Input: part model. Units: mm. Frame: model coordinates. Face numbers are marked on the shaded views. Round coordinates to 2 decimals unless told otherwise and drop trailing zeros. Write each loop counter-clockwise with the first axis right and the second up, starting at its lowest first coordinate (ties: lowest second). Pieces come first, ordered by that corner, then holes. Notation, with made-up numbers: M -32,65.25 L -15,65.25 A31 ccw -15,94.25 Z; hole C 39.5,11.25 d3. An arc over 180 degrees is marked long. Use one line per item in the form item = value. Start each with the question number.
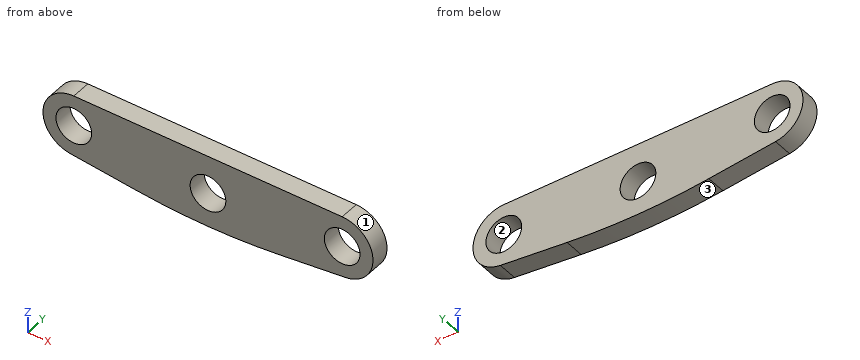
```python
from build123d import *

# Parameters (mm, degrees)
F0_R     = 5.5
F1_DEPTH = 6
F2_R     = 200


with BuildPart() as f1:
    # F0 (on Front) → F1 (new body)
    with BuildSketch(Plane.XZ):
        with BuildLine():
            Line((41.35, 11.8), (-41.35, 11.8))
            ThreePointArc((-41.35, 11.8), (-50.835785, 2.819506), (-42.387457, -7.143182))
            Line((-42.387457, -7.143182), (0, -11.8))
            Line((0, -11.8), (42.387457, -7.143182))
            ThreePointArc((42.387457, -7.143182), (50.835785, 2.819506), (41.35, 11.8))
        make_face()
        Circle(F0_R, mode=Mode.SUBTRACT)
        with Locations((-41.35, 2.3)):
            Circle(F0_R, mode=Mode.SUBTRACT)
        with Locations((41.35, 2.3)):
            Circle(F0_R, mode=Mode.SUBTRACT)
    extrude(amount=F1_DEPTH)

    # F2
    f2_edges = [f1.edges().sort_by_distance(p)[0] for p in [
        (0, -3, -11.8),
    ]]
    fillet(f2_edges, radius=F2_R)


solid = f1.part
```
Item 1: Cut plane C-C (y = -2.55). Output: boundary loops of the cut face in (x, z), plus the area to 3 significant figures.
Item 2: Cut plane D-D (z = 4.25). Output: boundary loops of the cut face in (x, y).
Item 3: Cut plane A-A (x = 0). Output: boundary loops of the cut face in (y, z).
Item 4: Draft query along X for the marked faces 1, 2 and 3. Return one class per face: +X half, -X half, draft (parallel to the pull), parting line (faces both ways), or undercut.
Item 5: Ray query, line 1 (Z direction, x = 0, y = -2.05); line 2 (X direction, y = -5.1, z = 5); line 3 (X direction, y = -2.8, z = 0.25). Return the intervals inside material, ascending. Write a range as from..to.
Item 6: Cut plane B-B (z = 0). Output: boundary loops of the cut face in (x, y).
Item 7: First-contact query: pin 1 (3 mm diameter, centred on x = 15, z = 6.5, fed in from +Y); pin 2 (6.5 mm diameter, centred on x = 41.35, z = 2.3, fed in from -Y); pin 3 (1.5 mm diameter, centred on x = 18.5, y = -4, fed in from -Z); pin 4 (1 mm diameter, centred on y = -1.5, z = 1.5, fed in from -X). Flat tips, straight axial feed; report the tip coordinate or a pass-through.
Final values:
q1.outline = M -42.39,-7.14 L -21.84,-9.4 A200 ccw 21.84,-9.4 L 42.39,-7.14 A9.5 ccw 41.35,11.8 L -41.35,11.8 A9.5 ccw Z; hole C -41.35,2.3 d11; hole C 0,0 d11; hole C 41.35,2.3 d11
q1.area = 1,740 mm^2
q2.outline = M -50.65,-6 L -46.49,-6 L -46.49,0 L -50.65,0 Z; M -36.21,-6 L -3.49,-6 L -3.49,0 L -36.21,0 Z; M 3.49,-6 L 36.21,-6 L 36.21,0 L 3.49,0 Z; M 46.49,-6 L 50.65,-6 L 50.65,0 L 46.49,0 Z
q3.outline = M -6,-10.6 L 0,-10.6 L 0,-5.5 L -6,-5.5 Z; M -6,5.5 L 0,5.5 L 0,11.8 L -6,11.8 Z
q4.face_1 = +X half
q4.face_2 = undercut
q4.face_3 = parting line
q5.line_1 = -10.6..-5.5, 5.5..11.8
q5.line_2 = -50.46..-46.14, -36.56..-2.29, 2.29..36.56, 46.14..50.46
q5.line_3 = -50.63..-46.45, -36.25..-5.49, 5.49..36.25, 46.45..50.63
q6.outline = M -50.57,-6 L -46.35,-6 L -46.35,0 L -50.57,0 Z; M -36.35,-6 L -5.5,-6 L -5.5,0 L -36.35,0 Z; M 5.5,-6 L 36.35,-6 L 36.35,0 L 5.5,0 Z; M 46.35,-6 L 50.57,-6 L 50.57,0 L 46.35,0 Z
q7.pin_1 = 0
q7.pin_2 = through
q7.pin_3 = -9.81
q7.pin_4 = -50.85
